Print and shaded views of the part. All mm, measured from the part's lowest x, y and z. A direction names the side the tool comes from. Round coordinates to 2 decimals unless told otherwise and drop trailing zeros. Loops run counter-clockwise (first coordinate to the right, second up) from the corner with the lowest first, then second, coordinate; pieces in that order, holes last. Notation, with made-up numbers: (40, -20) - (55, -20) arc R29 ccw to (55, 18) - close; hole circle Ø3 at (-5.75, 77). An arc over 180 degrees is marked (long way). Use one line per item in the form item = value.
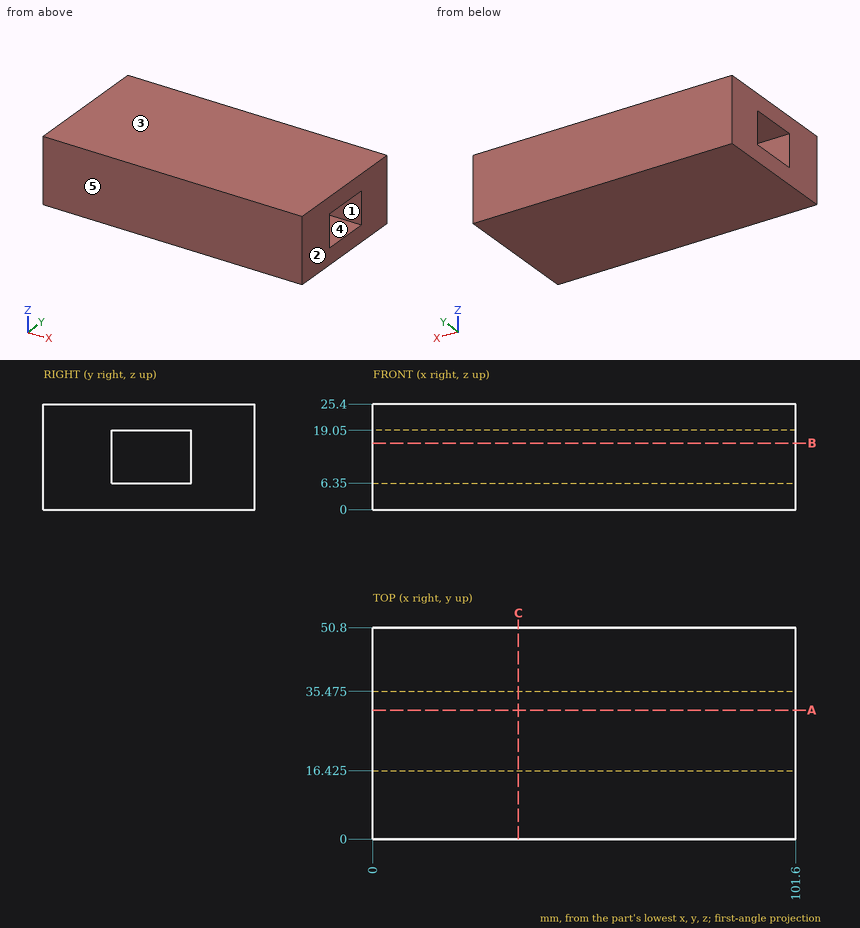
1) Tool access for the marked faces 1 and 2: list every direction of +Z, -Z, +X, -X, +Y, -Y with a clear straight run to the whole face (end or side of a thin tool).
Report:
face_1 = +X, -X
face_2 = +Z, -Z, +X, +Y, -Y
2) Two-plate mould, pull along Z, no slides. Class the marked faces 3, 4 and 5: +Z half, -Z half, draft (parallel to the pull), parting line (faces both ways), or undercut.
Report:
face_3 = +Z half
face_4 = undercut
face_5 = draft
3) Slice it at A-A (y = 31). Write the cut outline in (x, z).
Report:
outline = (0, 0) - (101.6, 0) - (101.6, 6.35) - (0, 6.35) - close; (0, 19.05) - (101.6, 19.05) - (101.6, 25.4) - (0, 25.4) - close
4) Drill centre lines: probe 1 along Y at (x, z) = (53.5, 12) (3 decimals); probe 2 along Z at (x, y) = (73, 24). Where is each one in solid material? Low to high.
Report:
probe_1 = 0 to 16.425, 35.475 to 50.8
probe_2 = 0 to 6.35, 19.05 to 25.4
5) Slice it at B-B (z = 16). Write the cut outline in (x, y) (3 decimals), plus the area to 3 significant figures.
Report:
outline = (0, 0) - (101.6, 0) - (101.6, 16.425) - (0, 16.425) - close; (0, 35.475) - (101.6, 35.475) - (101.6, 50.8) - (0, 50.8) - close
area = 3,230 mm^2
6) Slice it at C-C (x = 35). Write the cut outline in (y, z) (3 decimals), plus the area to 3 significant figures.
Report:
outline = (0, 0) - (50.8, 0) - (50.8, 25.4) - (0, 25.4) - close; hole (16.425, 6.35) - (35.475, 6.35) - (35.475, 19.05) - (16.425, 19.05) - close
area = 1,050 mm^2
